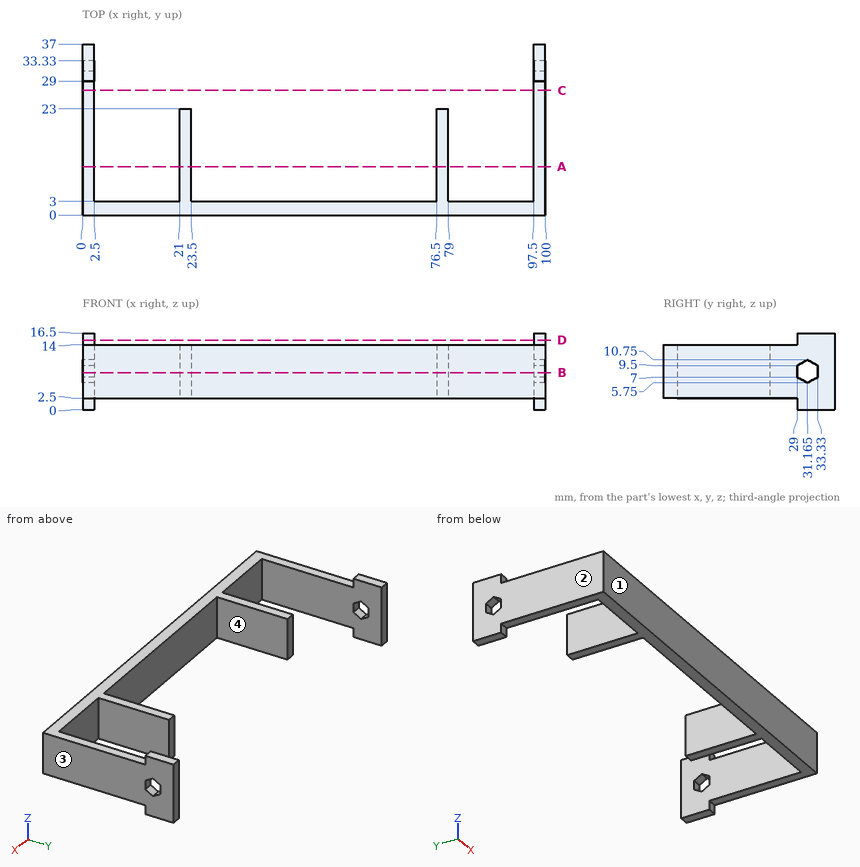
Geometry: see drawing. Coordinates: mm, zero at the bounding-box minimum. Round coordinates to 2 decimals unless told otherwise and drop trailing zeros. Write each loop counter-clockwise with the first axis right and the second up, starting at its lowest first coordinate (ties: lowest second). Pieces come first, ordered by that corner, then holes. Notation, with made-up numbers: M 6.5,55.25 L 13.5,55.25 A25 ccw 13.5,80.25 Z; hole C 71.25,16.5 d11. An arc over 180 degrees is marked long. Answer as a JSON object with one key per item and string values. Group by question number.
(1) Section query B-B on z = 8. Output: boundary loops of the cut face in (x, y), then the cut area to 3 significant figures.
(2) Section query D-D on z = 15. Output: boundary loops of the cut face in (x, y), then the cut area to 3 significant figures.
(3) Section query C-C on y = 27. Output: boundary loops of the cut face in (x, z).
(4) Mould query, pull axis X, two halves, no side actions, for the marked faces 1, 2, 3 and 4. Classes: +X half, -X half, draft (parallel to the pull), parting line (faces both ways), or undercut.
(5) Ray query, line 1 (X direction, y = 12.5, z = 12.25); line 2 (X direction, y = 35.5, z = 6.25); line 3 (Y direction, x = 57, z = 13). Return the intervals inside material, ascending. Write a range as [from, to].
(6) Section query A-A on y = 10.5. Output: boundary loops of the cut face in (x, z).
(7) First-contact query: pin 1 (1.2 mm diameter, centred on x = 21.5, z = 10, fed in from +Y); pin 2 (0.8 mm diameter, centred on x = 1, z = 15, fed in from -Y); pin 3 (3.5 mm diameter, centred on x = 88, z = 9.5, fed in from +Y). Flat tips, straight axial feed; report the tip coordinate or a pass-through.
Computed values:
{
 "1": {"outline": "M 0,0 L 100,0 L 100,29 L 97.5,29 L 97.5,3 L 79,3 L 79,23 L 76.5,23 L 76.5,3 L 23.5,3 L 23.5,23 L 21,23 L 21,3 L 2.5,3 L 2.5,29 L 0,29 Z; M 0,33.33 L 2.5,33.33 L 2.5,37 L 0,37 Z; M 97.5,33.33 L 100,33.33 L 100,37 L 97.5,37 Z", "area": "548 mm^2"},
 "2": {"outline": "M 0,29 L 2.5,29 L 2.5,37 L 0,37 Z; M 97.5,29 L 100,29 L 100,37 L 97.5,37 Z", "area": "40.0 mm^2"},
 "3": {"outline": "M 0,2.5 L 2.5,2.5 L 2.5,14 L 0,14 Z; M 97.5,2.5 L 100,2.5 L 100,14 L 97.5,14 Z"},
 "4": {"face 1": "draft", "face 2": "-X half", "face 3": "+X half", "face 4": "undercut"},
 "5": {"line 1": "[0, 2.5], [21, 23.5], [76.5, 79], [97.5, 100]", "line 2": "[0, 2.5], [97.5, 100]", "line 3": "[0, 3]"},
 "6": {"outline": "M 0,2.5 L 2.5,2.5 L 2.5,14 L 0,14 Z; M 21,2.5 L 23.5,2.5 L 23.5,14 L 21,14 Z; M 76.5,2.5 L 79,2.5 L 79,14 L 76.5,14 Z; M 97.5,2.5 L 100,2.5 L 100,14 L 97.5,14 Z"},
 "7": {"pin 1": "y = 23", "pin 2": "y = 29", "pin 3": "y = 3"}
}
